Work out the finished part from the listing and answer in its coordinate system (mm). Round coordinates to 2 decimals unless told otherwise and drop trailing zeros. Order: outer loops, then holes, each group sorted by start corner. A loop starts at its lowest first (then second) coordinate and runs counter-clockwise, first axis right, second up. Notation, with made-up numbers: (86.5, 16) -> (95.5, 16) arc R30 cw to (95.5, 48) -> close; hole circle Ø8 at (-32, 15.25). An arc over 180 degrees is marked (long way). Use one line per item in the form item = value.
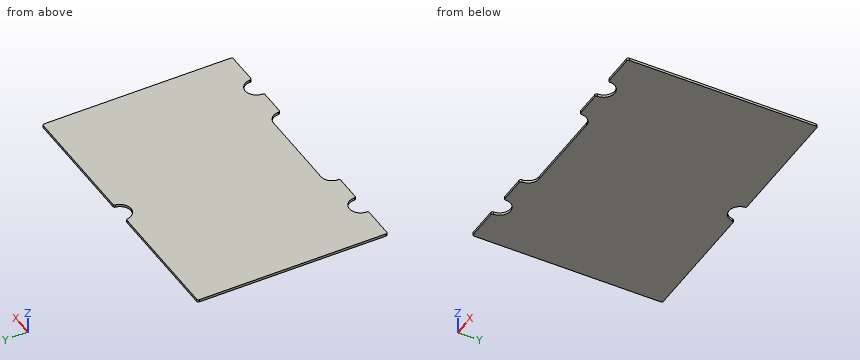
```python
from build123d import *

# Parameters (mm, degrees)
EXTRUDE_DEPTH = 1.5


with BuildPart() as part:
    # Sketch → Extrude (new body)
    with BuildSketch(Plane.XY):
        with BuildLine():
            Line((82, -55), (82, 55))
            ThreePointArc((82, 55), (81.707107, 55.707107), (81, 56))
            Line((81, 56), (7.433034, 56))
            ThreePointArc((7.433034, 56), (6.774754, 55.752773), (6.441963, 55.133333))
            ThreePointArc((0, 49.5), (4.278824, 51.106978), (6.441963, 55.133333))
            ThreePointArc((-6.441963, 55.133333), (-4.278824, 51.106978), (0, 49.5))
            ThreePointArc((-6.441963, 55.133333), (-6.774754, 55.752773), (-7.433034, 56))
            Line((-81, 56), (-7.433034, 56))
            ThreePointArc((-81, 56), (-81.707107, 55.707107), (-82, 55))
            Line((-82, -55), (-82, 55))
            ThreePointArc((-82, -55), (-81.707107, -55.707107), (-81, -56))
            Line((-62.5, -56), (-81, -56))
            ThreePointArc((-62.5, -56), (-61.792893, -55.707107), (-61.5, -55))
            ThreePointArc((-48.5, -55), (-55, -48.5), (-61.5, -55))
            ThreePointArc((-48.5, -55), (-48.207107, -55.707107), (-47.5, -56))
            Line((-32.5, -56), (-47.5, -56))
            ThreePointArc((-32.5, -56), (-31.792893, -55.707107), (-31.5, -55))
            ThreePointArc((-25, -48.5), (-29.596194, -50.403806), (-31.5, -55))
            Line((-25, -48.5), (0, -48.5))
            Line((25, -48.5), (0, -48.5))
            ThreePointArc((31.5, -55), (29.596194, -50.403806), (25, -48.5))
            ThreePointArc((31.5, -55), (31.792893, -55.707107), (32.5, -56))
            Line((32.5, -56), (47.5, -56))
            ThreePointArc((47.5, -56), (48.207107, -55.707107), (48.5, -55))
            ThreePointArc((61.5, -55), (55, -48.5), (48.5, -55))
            ThreePointArc((61.5, -55), (61.792893, -55.707107), (62.5, -56))
            Line((62.5, -56), (81, -56))
            ThreePointArc((81, -56), (81.707107, -55.707107), (82, -55))
        make_face()
    extrude(amount=EXTRUDE_DEPTH)


solid = part.part
```
Item 1: The part is cut by section A-A, the plane z = 1.15. Give the vertices of the cut face in (x, y).
Findings:
outline = (-82, -55) arc R1 ccw to (-81, -56) -> (-62.5, -56) arc R1 ccw to (-61.5, -55) arc R6.5 cw to (-48.5, -55) arc R1 ccw to (-47.5, -56) -> (-32.5, -56) arc R1 ccw to (-31.5, -55) arc R6.5 cw to (-25, -48.5) -> (25, -48.5) arc R6.5 cw to (31.5, -55) arc R1 ccw to (32.5, -56) -> (47.5, -56) arc R1 ccw to (48.5, -55) arc R6.5 cw to (61.5, -55) arc R1 ccw to (62.5, -56) -> (81, -56) arc R1 ccw to (82, -55) -> (82, 55) arc R1 ccw to (81, 56) -> (7.43, 56) arc R1 ccw to (6.44, 55.13) arc R6.5 cw to (-6.44, 55.13) arc R1 ccw to (-7.43, 56) -> (-81, 56) arc R1 ccw to (-82, 55) -> close
Item 2: A flat-ended cylindrical pin translates along its axis: P1, Ø0.8, axis at x = 10, z = 1, coming from the -Y side. Find the tip coordinate at first contact, or state that the pin passes through.
Findings:
P1 = -48.5
Item 3: The part is cut by section B-B, the plane x = -55. Give the vertices of the cut face in (y, z).
Findings:
outline = (-48.5, 0) -> (56, 0) -> (56, 1.5) -> (-48.5, 1.5) -> close
Item 4: Consider line 1 along X through (y, z) = (-49, 0.45); line 2 along Y through (x, z) = (11, 1.1); line 3 along X through (y, z) = (51, 1.25). Determine where each line is inside the solid, lowest interval first.
Findings:
line_1 = -82 to -57.5, -52.5 to -27.5, 27.5 to 52.5, 57.5 to 82
line_2 = -48.5 to 56
line_3 = -82 to -4.15, 4.15 to 82
